Source: CAD feature listing. Evaluate the final solid. Frame: model axes, mm. A direction names the side the tool comes from. Give positions to 0.01 mm unless a question says otherwise; leave off trailing zeros. Write each loop counter-clockwise with the first axis right and the second up, starting at its lowest first coordinate (ties: lowest second). Pieces come first, ordered by that corner, then holes. Notation, with made-up numbers: (57.25, 17.25) - (68.25, 17.25) arc R21 ccw to (68.25, 23.25) - close; hole circle Ø5 at (-33, 20). An arc over 180 degrees is marked (long way). One line per question, with ' | ' between items. Start each with the question number.
(1) Access query for faces 1 (the flat face through (86, 170, 5)), 2 (the flat face through (80.906, 77.368, 5.07)), 3 (the flat face through (150, 55, 5)). Directions: +Z, -Z, +X, -X, +Y, -Y. A direction counts if a zero-diameter tool reaches every point of the face in a straight line with its end or side. Return the directions, or none.
(2) Draft query along X for faces 4 (the flat face through (170, 27, 5)), 5 (the flat face through (80.437, 92.361, 5.07)), 6 (the flat face through (65, 86, 0)). Return one class per face: +X half, -X half, draft (parallel to the pull), parting line (faces both ways), or undercut.
(3) Ray query, line 1 (Y direction, x = 15, z = 6); line 2 (Y direction, x = 154.5, z = 7.75). Return the intervals inside material, ascending. Write a range as [from, to].
(4) Section A-A, the plane y = 15. Return loops of the section in (x, z), plus the area to 3 significant figures.
(5) Section C-C, the plane z = 8.5. Return loops of the section in (x, y).
(6) Section D-D, the plane x = 115. Return loops of the section in (y, z).
(7) Section B-B, the plane x = 155. Return loops of the section in (y, z).
(8) Pin query (flat end, axial travel): pin 1 (1 mm diameter, centred on y = 107.5, z = 4.5, fed in from +X). Return the tip coordinate at first contact, or that it passes through.
Autodesk Inventor part; units mm, degrees
ref_plane "YZ Plane" through (0, 0, 0) normal (1, 0, 0) x (0, 1, 0)
ref_plane "XZ Plane" through (0, 0, 0) normal (0, 1, 0) x (-1, 0, 0)
ref_plane "XY Plane" through (0, 0, 0) normal (0, 0, 1) x (1, 0, 0)
sketch "Sketch1" plane through (0, 0, 0) normal (0, 0, 1) x (1, 0, 0)
  line L0 (0, 0) -> (170, 0)
  line L1 (170, 0) -> (170, 170)
  line L2 (170, 170) -> (0, 170)
  line L3 (0, 170) -> (0, 0)
  dimension "d0" = 170
  dimension "d1" = 170
extrude "Extrusion1" add sketch "Sketch1" along normal blind 10
sketch "Sketch2" plane through (0, 0, 10) normal (0, 0, 1) x (1, 0, 0)
  line L0 (170, 170) -> (0, 170)
  line L1 (0, 170) -> (0, 155)
  line L2 (0, 170) -> (0, 0)
  line L3 (0, 0) -> (170, 0)
  line L4 (0, 0) -> (0, 15)
  line L5 (0, 15) -> (155, 15)
  line L6 (155, 15) -> (155, 155)
  line L7 (155, 155) -> (15, 155)
  line L8 (15, 155) -> (15, 15)
  line L9 (15, 155) -> (30, 155)
  circle A0 centre (15, 155) radius 7.5
  circle A1 centre (155, 155) radius 7.5
  circle A2 centre (155, 15) radius 7.5
  circle A3 centre (15, 15) radius 7.5
  dimension "d4" = 15
  dimension "d5" = 15
  dimension "d6" = 155
  dimension "d7" = 140
  dimension "d8" = 140
  dimension "d9" = 140
  dimension "d10" = 15
  dimension "d11" = 15
  dimension "d12" = 15
  dimension "d13" = 15
extrude "Extrusion2" cut sketch "Sketch2" against normal blind 10 contours L8 A3 L5 | L5 A3 | L5 A3 L8 | A2 L6 L5 | L5 L6 A2 | A0 L7 L8 | L8 L7 A0 | A1 L7 L6 | L6 L7 A1
sketch "Sketch3" plane through (0, 0, 10) normal (0, 0, 1) x (1, 0, 0)
  line L0 (170, 170) -> (0, 170)
  line L1 (0, 170) -> (85, 170)
  line L2 (85, 170) -> (85, 85)
  line L3 (93.542, 90.1995) -> (93.7739, 80.2022)
  line L4 (93.7739, 80.2022) -> (85.2319, 75.0027)
  line L5 (85.2319, 75.0027) -> (76.458, 79.8005)
  line L6 (76.458, 79.8005) -> (76.2261, 89.7978)
  line L7 (76.2261, 89.7978) -> (84.7681, 94.9973)
  line L8 (84.7681, 94.9973) -> (93.542, 90.1995)
  point P0 (0, 0)
  dimension "d16" = 85
  dimension "d17" = 85
  dimension "d18" = 10
extrude "Extrusion3" cut sketch "Sketch3" against normal blind 10
sketch "Sketch4" plane through (0, 0, 10) normal (0, 0, 1) x (1, 0, 0)
  line L0 (170, 170) -> (0, 170)
  line L1 (0, 170) -> (85, 170)
  line L2 (85, 170) -> (85, 150)
  line L3 (85, 150) -> (85, 20)
  circle A0 centre (85, 150) radius 2.5
  circle A1 centre (85, 20) radius 2.5
  point P0 (0, 0)
  dimension "d21" = 85
  dimension "d22" = 20
  dimension "d23" = 130
  dimension "d24" = 5
  dimension "d25" = 5
extrude "Extrusion4" cut sketch "Sketch4" against normal blind 10
sketch "Sketch5" plane through (0, 0, 10) normal (0, 0, 1) x (1, 0, 0)
  line L0 (170, 170) -> (0, 170)
  line L1 (170, 170) -> (170, 85)
  line L2 (170, 0) -> (170, 170)
  point P0 (0, 0)
  dimension "d28" = 85
sketch "Sketch6" plane through (0, 0, 10) normal (0, 0, 1) x (1, 0, 0)
  line L0 (170, 0) -> (170, 170)
  line L1 (170, 85) -> (130, 85)
  circle A0 centre (130, 85) radius 30
  point P0 (0, 0)
  dimension "d29" = 40
  dimension "d30" = 60
extrude "Extrusion5" cut sketch "Sketch6" against normal blind 10
sketch "Sketch7" plane through (0, 0, 10) normal (0, 0, 1) x (1, 0, 0)
  line L0 (170, 0) -> (170, 170)
  line L1 (170, 85) -> (170, 55)
  line L2 (170, 55) -> (170, 115)
  line L3 (170, 115) -> (157, 115)
  line L4 (157, 115) -> (157, 55)
  line L5 (157, 55) -> (170, 55)
  line L6 (170, 55) -> (170, 115)
  point P0 (0, 0)
  dimension "d33" = 30
  dimension "d34" = 60
extrude "Extrusion6" cut sketch "Sketch7" against normal blind 10
sketch "Sketch8" plane through (0, 0, 10) normal (0, 0, 1) x (1, 0, 0)
  line L0 (157, 55) -> (157, 71.9233)
  line L1 (157, 55) -> (138, 55)
  line L2 (138, 55) -> (130, 55)
  arc A0 (157, 98.0767) -> (157, 71.9233) centre (130, 85) ccw
  point P0 (0, 0)
extrude "Extrusion7" cut sketch "Sketch8" against normal blind 10
sketch "Sketch9" plane through (0, 0, 10) normal (0, 0, 1) x (1, 0, 0)
  line L0 (157, 115) -> (157, 98.0767)
  line L1 (157, 115) -> (130, 115)
  arc A0 (157, 98.0767) -> (130, 55) centre (130, 85) ccw
  point P0 (0, 0)
extrude "Extrusion8" cut sketch "Sketch9" against normal blind 10
properties part number "AC"
Check sheet entries:
1) face 1: +Z, -Z, +X, -X, +Y | face 2: +Z, -Z | face 3: +Z, -Z, +X
2) face 4: +X half | face 5: undercut | face 6: draft
3) line 1: [0, 7.5], [22.5, 147.5], [162.5, 170] | line 2: [0, 7.52], [22.48, 55], [115, 147.52], [162.48, 170]
4) outline: (0, 0) - (7.5, 0) - (7.5, 10) - (0, 10) - close; (22.5, 0) - (147.5, 0) - (147.5, 10) - (22.5, 10) - close; (162.5, 0) - (170, 0) - (170, 10) - (162.5, 10) - close | area: 1,400 mm²
5) outline: (0, 0) - (170, 0) - (170, 55) - (130, 55) arc R30 cw to (130, 115) - (170, 115) - (170, 170) - (0, 170) - close; hole circle Ø15 at (15, 15); hole circle Ø15 at (15, 155); hole (76.23, 89.8) - (76.46, 79.8) - (85.23, 75) - (93.77, 80.2) - (93.54, 90.2) - (84.77, 95) - close; hole circle Ø5 at (85, 20); hole circle Ø5 at (85, 150); hole circle Ø15 at (155, 15); hole circle Ø15 at (155, 155)
6) outline: (0, 0) - (59.02, 0) - (59.02, 10) - (0, 10) - close; (110.98, 0) - (170, 0) - (170, 10) - (110.98, 10) - close
7) outline: (0, 0) - (7.5, 0) - (7.5, 10) - (0, 10) - close; (22.5, 0) - (55, 0) - (55, 10) - (22.5, 10) - close; (115, 0) - (147.5, 0) - (147.5, 10) - (115, 10) - close; (162.5, 0) - (170, 0) - (170, 10) - (162.5, 10) - close
8) pin 1: x = 110.74
